from build123d import *

# Parameters (mm, degrees)
MODEL_W                 = 10
MODEL_H                 = 2.9
SALIENTE_EXTRUIR1_DEPTH = 0.1


with BuildPart() as part:
    # Model → Saliente-Extruir1 (new body)
    with BuildSketch(Plane.XY):
        with BuildLine():
            Line((35.788328911, 21.707483708), (34.562799173, 21.581308157))
            Line((34.562799173, 21.581308157), (34.562652828, 22.581308147))
            Line((34.562652828, 22.581308147), (32.70612679, 23.481266233))
            Line((32.70612679, 23.481266233), (32.556235076, 26.619326304))
            Line((32.556235076, 26.619326304), (31.036614796, 27.404548337))
            ThreePointArc((31.036614796, 27.404548337), (32.854753025, 46.472842043), (31.55872141, 65.583722544))
            ThreePointArc((31.55872141, 65.583722544), (30.590969531, 65.595574241), (29.845859092, 64.977921752))
            ThreePointArc((29.845859092, 64.977921752), (29.533169752, 62.324588377), (29.332558898, 59.660435997))
            ThreePointArc((29.332558898, 59.660435997), (29.087424273, 55.159098423), (28.459158768, 50.695085274))
            ThreePointArc((28.459158768, 50.695085274), (28.627310402, 45.667965845), (28.027763798, 40.673894501))
            Line((28.027763798, 40.673894501), (22.450336553, 41.621102944))
            ThreePointArc((22.450336553, 41.621102944), (22.785375557, 45.632918576), (23.55872141, 49.583722544))
            ThreePointArc((23.55872141, 49.583722544), (22.508827615, 59.842451026), (23.202312308, 70.131419197))
            ThreePointArc((23.202312308, 70.131419197), (24.161095869, 72.639029062), (25.666362665, 74.861987681))
            ThreePointArc((25.666362665, 74.861987681), (26.473042164, 75.27855447), (27.341750173, 75.542384144))
            Line((27.341750173, 75.542384144), (27.561102277, 75.584512547))
            Line((27.561102277, 75.584512547), (30.155444554, 75.902266174))
            Line((30.155444554, 75.902266174), (40.23046228, 76.952955231))
            ThreePointArc((40.23046228, 76.952955231), (41.577753061, 73.95916021), (44.55872141, 72.583722544))
            Line((44.55872141, 72.583722544), (48.101813752, 64.261756561))
            Line((48.101813752, 64.261756561), (35.059978867, 64.261756561))
            Line((35.059978867, 64.261756561), (35.059978867, 32.261756561))
            Line((35.059978867, 32.261756561), (67.059978867, 32.261756561))
            Line((67.059978867, 32.261756561), (67.059978867, 64.261756561))
            Line((67.059978867, 64.261756561), (54.018143983, 64.261756561))
            Line((54.018143983, 64.261756561), (57.561236324, 72.583722544))
            ThreePointArc((57.561236324, 72.583722544), (60.537265907, 73.954182145), (61.888562624, 76.938961663))
            Line((61.888562624, 76.938961663), (73.033030733, 75.731471954))
            ThreePointArc((73.033030733, 75.731471954), (74.577070762, 75.460810441), (76.095189277, 75.070127146))
            ThreePointArc((76.095189277, 75.070127146), (77.804128562, 73.593895905), (78.689246297, 71.516325509))
            ThreePointArc((78.689246297, 71.516325509), (79.299082123, 66.847407918), (79.563217831, 62.146245983))
            ThreePointArc((79.563217831, 62.146245983), (79.348252658, 55.842170985), (78.561236324, 49.583722544))
            ThreePointArc((78.561236324, 49.583722544), (79.338265829, 45.606384219), (79.67109964, 41.567545691))
            Line((79.67109964, 41.567545691), (74.092351811, 40.669243886))
            ThreePointArc((74.092351811, 40.669243886), (73.494321928, 45.665313622), (73.659828166, 50.694325476))
            ThreePointArc((73.659828166, 50.694325476), (73.032031827, 55.158739267), (72.787398837, 59.660435997))
            ThreePointArc((72.787398837, 59.660435997), (72.586787983, 62.324588377), (72.274098643, 64.977921752))
            ThreePointArc((72.274098643, 64.977921752), (71.528988204, 65.595574241), (70.561236324, 65.583722544))
            ThreePointArc((70.561236324, 65.583722544), (69.272286317, 46.443233149), (71.102210852, 27.346869554))
            ThreePointArc((71.102210852, 27.346869554), (70.310817444, 27.032315031), (69.5645482, 26.622034286))
            Line((69.5645482, 26.622034286), (69.415115725, 23.483952313))
            Line((69.415115725, 23.483952313), (67.55872141, 22.583722544))
            Line((67.55872141, 22.583722544), (67.55872141, 21.583722544))
            Line((67.55872141, 21.583722544), (66.33317322, 21.709718743))
            ThreePointArc((66.33317322, 21.709718743), (60.608385736, 21.918148973), (55.064572652, 20.474967974))
            ThreePointArc((55.064572652, 20.474967974), (51.060864546, 20.157739519), (47.057110058, 20.47438205))
            ThreePointArc((47.057110058, 20.47438205), (41.513085831, 21.916751726), (35.788328911, 21.707483708))
        make_face()
        with Locations((58.559978867, 26.033722544)):
            Rectangle(MODEL_W, MODEL_H, mode=Mode.SUBTRACT)
        with Locations((43.559978867, 26.033722544)):
            Rectangle(MODEL_W, MODEL_H, mode=Mode.SUBTRACT)
    extrude(amount=SALIENTE_EXTRUIR1_DEPTH)


solid = part.part
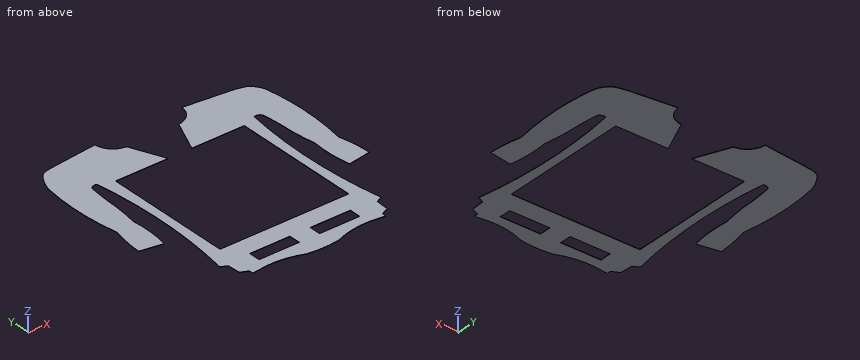
Check sheet for the modelled part. Datum: model origin and axes. Units: mm. Round coordinates to 2 decimals unless told otherwise and drop trailing zeros. Loops run counter-clockwise (first coordinate to the right, second up) from the corner with the lowest first, then second, coordinate; pieces in that order, holes last.
1. Sectioned sample at A-A on x = 42.5. Record the boundary of the cut face in (y, z), and give its area (3 significant figures).
2. Sectioned sample at D-D on x = 59.5. Record the boundary of the cut face in (y, z).
3. Sectioned sample at C-C on y = 47. Record the boundary of the cut face in (x, z).
4. Scan lines: probe 1 along Y at (x, z) = (37, 0.05); probe 2 along Y at (x, z) = (30, 0.05). Record each from-to range of solid material in increasing order.
5. Gauge pin test, flat end, axial feed: pin 1 Ø1 at (x, y) = (35, 43) entering from -Z. Record the tip position at first contact, or that the pin passes through.
6. Sectioned sample at B-B on y = 37. Record the boundary of the cut face in (x, z), and give its area (3 significant figures).
Recorded:
1. outline: (21.78, 0) - (24.58, 0) - (24.58, 0.1) - (21.78, 0.1) - close; (27.48, 0) - (32.26, 0) - (32.26, 0.1) - (27.48, 0.1) - close; (64.26, 0) - (73.24, 0) - (73.24, 0.1) - (64.26, 0.1) - close
1. area: 1.66 mm2
2. outline: (21.76, 0) - (24.58, 0) - (24.58, 0.1) - (21.76, 0.1) - close; (27.48, 0) - (32.26, 0) - (32.26, 0.1) - (27.48, 0.1) - close; (64.26, 0) - (73.17, 0) - (73.17, 0.1) - (64.26, 0.1) - close
3. outline: (23, 0) - (28.66, 0) - (28.66, 0.1) - (23, 0.1) - close; (32.86, 0) - (35.06, 0) - (35.06, 0.1) - (32.86, 0.1) - close; (67.06, 0) - (69.27, 0) - (69.27, 0.1) - (67.06, 0.1) - close; (73.46, 0) - (79.12, 0) - (79.12, 0.1) - (73.46, 0.1) - close
4. probe 1: y = 21.89 to 32.26, 64.26 to 76.62
4. probe 2: y = 65.19 to 75.88
5. pin 1: stops at z = 0
6. outline: (32.34, 0) - (35.06, 0) - (35.06, 0.1) - (32.34, 0.1) - close; (67.06, 0) - (69.78, 0) - (69.78, 0.1) - (67.06, 0.1) - close
6. area: 0.544 mm2
